The listing builds one solid part. Answer for the finished solid, in the listing's coordinates (mm). A direction names the side the tool comes from. Give positions to 0.01 mm unless a question says otherwise; leave off trailing zeros. Loops run counter-clockwise (first coordinate to the right, second up) from the corner with the lowest first, then second, coordinate; pieces in that order, holes last. Notation, with made-up numbers: M 1.5,67.5 L 45.5,67.5 A22 cw 45.5,86.5 Z; hole C -28.5,7.5 d10. An arc over 180 degrees is marked long. Return JSON: item names as keys, results as strings.
from build123d import *

# Parameters (mm, degrees)
SKETCH1_R           = 7.5
SKETCH1_R_2         = 4
BOSS_EXTRUDE1_DEPTH = 10
SKETCH2_R           = 7
BOSS_EXTRUDE2_DEPTH = 1
BOSS_EXTRUDE3_START = 1
SKETCH3_R           = 7
BOSS_EXTRUDE3_DEPTH = 1
BOSS_EXTRUDE4_START = 2.5
SKETCH5_R           = 7.5
BOSS_EXTRUDE4_DEPTH = 2.5
SKETCH10_W          = 1
SKETCH10_H          = 12
CUT_EXTRUDE4_DEPTH  = 10
SKETCH11_W          = 12
SKETCH11_H          = 1
CUT_EXTRUDE5_DEPTH  = 10
SKETCH6_R           = 7.5
BOSS_EXTRUDE6_DEPTH = 2.5
CUT_EXTRUDE1_START  = -17
SKETCH7_R           = 4
CUT_EXTRUDE1_DEPTH  = 17
SKETCH8_R           = 6.75
SKETCH8_R_2         = 4.75
CUT_EXTRUDE2_DEPTH  = 0.1
CUT_EXTRUDE3_START  = -0.1
SKETCH9_R           = 6.75
SKETCH9_R_2         = 4.75
CUT_EXTRUDE3_DEPTH  = 0.1


with BuildPart() as part:
    # Sketch1 → Boss-Extrude1 (new body)
    with BuildSketch(Plane.XY):
        Circle(SKETCH1_R)
        Circle(SKETCH1_R_2, mode=Mode.SUBTRACT)
    extrude(amount=BOSS_EXTRUDE1_DEPTH)

    # Sketch2 → Boss-Extrude2 (add)
    with BuildSketch(Plane.XY.offset(10)):
        Circle(SKETCH2_R)
    extrude(amount=BOSS_EXTRUDE2_DEPTH)

    # Sketch3 → Boss-Extrude3 (add)
    with BuildSketch(Plane(origin=(0, 0, 0), x_dir=(-1, 0, 0), z_dir=(0, 0, -1)).offset(BOSS_EXTRUDE3_START)):
        with Locations(Location((0, 0, 0), (0, 0, 180))):
            Circle(SKETCH3_R)
    extrude(amount=-BOSS_EXTRUDE3_DEPTH)

    # Sketch5 → Boss-Extrude4 (add)
    with BuildSketch(Plane(origin=(0, 0, -1), x_dir=(-1, 0, 0), z_dir=(0, 0, -1)).offset(BOSS_EXTRUDE4_START)):
        with Locations(Location((0, 0, 0), (0, 0, 180))):
            Circle(SKETCH5_R)
    extrude(amount=-BOSS_EXTRUDE4_DEPTH)

    # Sketch10 → Cut-Extrude4 (cut)
    with BuildSketch(Plane.XY.offset(11)):
        Rectangle(SKETCH10_W, SKETCH10_H)
    extrude(amount=-CUT_EXTRUDE4_DEPTH, mode=Mode.SUBTRACT)

    # Sketch11 → Cut-Extrude5 (cut)
    with BuildSketch(Plane.XY.offset(11)):
        Rectangle(SKETCH11_W, SKETCH11_H)
    extrude(amount=-CUT_EXTRUDE5_DEPTH, mode=Mode.SUBTRACT)

    # Sketch6 → Boss-Extrude6 (add)
    with BuildSketch(Plane.XY.offset(11)):
        Circle(SKETCH6_R)
    extrude(amount=BOSS_EXTRUDE6_DEPTH)

    # Sketch7 → Cut-Extrude1 (cut)
    with BuildSketch(Plane.XY.offset(13.5).offset(CUT_EXTRUDE1_START)):
        Circle(SKETCH7_R)
    extrude(amount=CUT_EXTRUDE1_DEPTH, mode=Mode.SUBTRACT)

    # Sketch8 → Cut-Extrude2 (cut)
    with BuildSketch(Plane.XY.offset(13.5)):
        Circle(SKETCH8_R)
        Circle(SKETCH8_R_2, mode=Mode.SUBTRACT)
    extrude(amount=-CUT_EXTRUDE2_DEPTH, mode=Mode.SUBTRACT)

    # Sketch9 → Cut-Extrude3 (cut)
    with BuildSketch(Plane(origin=(0, 0, -3.5), x_dir=(-1, 0, 0), z_dir=(0, 0, -1)).offset(CUT_EXTRUDE3_START)):
        with Locations(Location((0, 0, 0), (0, 0, 180))):
            Circle(SKETCH9_R)
        with Locations(Location((0, 0, 0), (0, 0, 180))):
            Circle(SKETCH9_R_2, mode=Mode.SUBTRACT)
    extrude(amount=CUT_EXTRUDE3_DEPTH, mode=Mode.SUBTRACT)


solid = part.part
(1) Determine the mould class of faces 1 (the flat face through (-7, 1, 13.5)), 2 (the flat face through (0.5, -5, 6)), 3 (the cylindrical face through (4.032, -6.324, -2.268)) for opening direction Y: released by +Y, released by -Y, zero draft, split by the parting line, or undercut.
Values follow:
{"face 1": "zero draft", "face 2": "undercut", "face 3": "split by the parting line"}
(2) Straight lines are drawn through the part: line 1 along Z through (x, y) = (5.5, 4.75); line 2 along Y through (x, z) = (0, 3); line 3 along Z through (x, y) = (0.25, -5.5). For each, find the intervals that lie inside material, in ascending order.
Values follow:
{"line 1": "-3.5 to -1, 0 to 10, 11 to 13.5", "line 2": "-7.5 to -6, 6 to 7.5", "line 3": "-3.4 to 1, 11 to 13.4"}
(3) Given pin 1 (2 mm diameter, centred on x = -6, z = 9, fed in from -Y); pin 2 (0.6 mm diameter, centred on y = -5, z = 6, fed in from +X); pin 3 (1 mm diameter, centred on y = -4.5, z = 5.5, fed in from +X); pin 4 (9 mm diameter, centred on x = 0, y = 0, fed in from -Z), each flat-ended and moving along its own axis, determine where each tip first touches the part or whether it passes through.
Values follow:
{"pin 1": "y = -5.59", "pin 2": "x = 5.84", "pin 3": "x = 6.34", "pin 4": "z = -3.5"}
(4) The part is cut by section C-C (y = 6.25). Determine the outline of the cut face in (x, z), and give its area (3 significant figures).
Values follow:
{"outline": "M -4.15,-3.5 L -2.55,-3.5 L -2.55,-3.4 L 2.55,-3.4 L 2.55,-3.5 L 4.15,-3.5 L 4.15,-1 L 3.15,-1 L 3.15,0 L 4.15,0 L 4.15,10 L 3.15,10 L 3.15,11 L 4.15,11 L 4.15,13.5 L 2.55,13.5 L 2.55,13.4 L -2.55,13.4 L -2.55,13.5 L -4.15,13.5 L -4.15,11 L -3.15,11 L -3.15,10 L -4.15,10 L -4.15,0 L -3.15,0 L -3.15,-1 L -4.15,-1 Z", "area": "136 mm²"}
(5) A tool of negligible diameter and unlimited length cuts with its end or side. For faces 4 (the flat face through (1, 5, 13.4)), 5 (the flat face through (-5, -0.5, 6)), 6 (the cylindrical face through (-7.493, 0.33, 4.93)), from which of +Z, -Z, +X, -X, +Y, -Y can it reach the whole face along a straight path? Write none if from no direction.
Values follow:
{"face 4": "+Z", "face 5": "none", "face 6": "+Z, -Z"}
(6) The part is cut by section A-A (z = 9.5). Determine the outline of the cut face in (x, y).
Values follow:
{"outline": "C 0,0 d15; hole M -6,-0.5 L -3.97,-0.5 A4 ccw -0.5,-3.97 L -0.5,-6 L 0.5,-6 L 0.5,-3.97 A4 ccw 3.97,-0.5 L 6,-0.5 L 6,0.5 L 3.97,0.5 A4 ccw 0.5,3.97 L 0.5,6 L -0.5,6 L -0.5,3.97 A4 ccw -3.97,0.5 L -6,0.5 Z"}
